Build history of the part. All positions in model axes, mm. Face numbers are marked on the shaded views. A direction names the side the tool comes from. Give positions to 0.01 mm unless a question says otherwise; leave off trailing zeros. Loops run counter-clockwise (first coordinate to the right, second up) from the corner with the lowest first, then second, coordinate; pieces in that order, holes last. Notation, with made-up numbers: (83.25, 73.5) -> (90.25, 73.5) arc R23 cw to (90.25, 104.5) -> close; hole circle Ø11 at (59.5, 84.25). An arc over 180 degrees is marked (long way). Answer as a JSON object with one key per item and string values. Group by question number.
Q1. Two-plate mould, pull along Y, no slides. Class the marked faces 1, 2, 3 and 4: pulls with the +Y half, pulls with the -Y half, needs draft (parallel to the pull), parting line crosses it, or undercut.
Q2. Wall check: probe 1 along Y at (x, z) = (86, 89.5); probe 2 along Y at (x, z) = (105, 38); probe 3 along X at (y, z) = (-14, 48). Give the ranges that are in metal, low to high. Write a range as from..to.
Q3. Band-saw the part on B-B, the plane x = 8.5. Write the cut outline in (y, z), plus the area to 3 significant figures.
Q4. Band-saw the part on A-A, the plane y = 41. Write the cut outline in (x, z), plus the area to 3 significant figures.
Q5. Band-saw the part on C-C, the plane z = 78.5. Write the cut outline in (x, y).
Q6. Drop flat-ended pins along their axis: pin 1 (3 mm diameter, centred on y = -104.5, z = 61, fed in from -X); pin 2 (1 mm diameter, centred on x = -57, z = 21, fed in from +Y); pin 3 (1.5 mm diameter, centred on x = -72, y = -72, fed in from +Z). Give the stop position or say it passes through.
Q7. Band-saw the part on D-D, the plane z = 14. Write the cut outline in (x, y).
Q8. Tool access for the marked faces 5 and 6: list every direction of +Z, -Z, +X, -X, +Y, -Y with a clear straight run to the whole face (end or side of a thin tool).
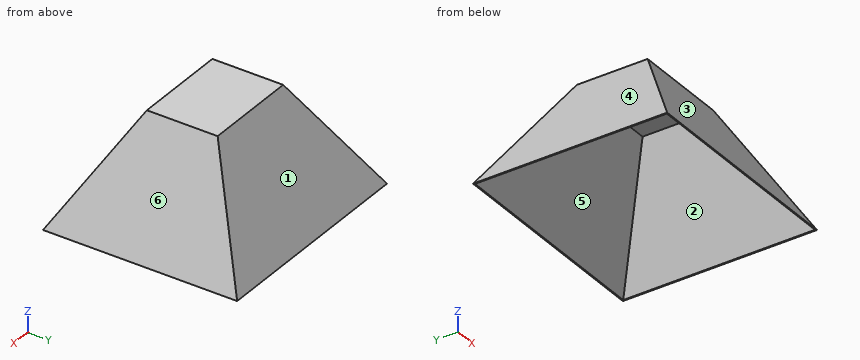
from build123d import *

# Parameters (mm, degrees)
SKETCH1_W           = 350
SKETCH1_H           = 310
BOSS_EXTRUDE1_DEPTH = 170.6
BOSS_EXTRUDE1_TAPER = 30
SHELL1_T            = -1.67


with BuildPart() as part:
    # Sketch1 → Boss-Extrude1 (new body)
    with BuildSketch(Plane.XY):
        Rectangle(SKETCH1_W, SKETCH1_H)
    extrude(amount=BOSS_EXTRUDE1_DEPTH, taper=BOSS_EXTRUDE1_TAPER)

    # Shell1
    shell1_openings = [part.faces().sort_by_distance(p)[0] for p in [
        (0, 0, 0),
    ]]
    offset(amount=SHELL1_T, openings=shell1_openings, kind=Kind.INTERSECTION)


solid = part.part
Worked answers:
{
 "1": {"face 1": "pulls with the +Y half", "face 2": "undercut", "face 3": "pulls with the -Y half", "face 4": "needs draft"},
 "2": {"probe 1": "-103.33..-101.4, 101.4..103.33", "probe 2": "-133.06..-131.13, 131.13..133.06", "probe 3": "-147.29..-145.36, 145.36..147.29"},
 "3": {"outline": "(-155, 0) -> (-153.07, 0) -> (-55.54, 168.93) -> (55.54, 168.93) -> (153.07, 0) -> (155, 0) -> (56.5, 170.6) -> (-56.5, 170.6) -> close", "area": "842 mm2"},
 "4": {"outline": "(-175, 0) -> (-173.07, 0) -> (-75.54, 168.93) -> (75.54, 168.93) -> (173.07, 0) -> (175, 0) -> (76.5, 170.6) -> (-76.5, 170.6) -> close", "area": "909 mm2"},
 "5": {"outline": "(-129.68, -109.68) -> (129.68, -109.68) -> (129.68, 109.68) -> (-129.68, 109.68) -> close; hole (-127.75, -107.75) -> (127.75, -107.75) -> (127.75, 107.75) -> (-127.75, 107.75) -> close"},
 "6": {"pin 1": "x = -140.65", "pin 2": "y = 143.16", "pin 3": "z = 145.06"},
 "7": {"outline": "(-166.92, -146.92) -> (166.92, -146.92) -> (166.92, 146.92) -> (-166.92, 146.92) -> close; hole (-164.99, -144.99) -> (164.99, -144.99) -> (164.99, 144.99) -> (-164.99, 144.99) -> close"},
 "8": {"face 5": "-Z", "face 6": "+Z, +X, +Y, -Y"}
}
